from build123d import *

# Parameters (mm, degrees)
F1_DEPTH = 6.35
F2_DEPTH = 12.7


with BuildPart() as f1:
    # F0 (on Front) → F1 (new body)
    with BuildSketch(Plane.XZ):
        Polygon((-29.3310899078, 53.6682253753), (-52.3154214025, 53.6682253753), (-52.3154214025, -22.5317746247), (54.824039946, -22.5317746247), (54.824039946, -8.9082447812), (44.4758199155, -8.9082447812), (44.4758199155, -2.3659907747), (54.824039946, -2.3659907747), (54.824039946, 13.8338748366), (44.4758199155, 13.8338748366), (44.4758199155, 21.3107354939), (54.824039946, 21.3107354939), (54.824039946, 36.2644605339), (44.4758199155, 36.2644605339), (44.4758199155, 44.3643927574), (54.824039946, 44.3643927574), (54.824039946, 55.1141475241), (31.8397084513, 54.8039578557), (-29.3310899078, 53.9784150436), align=None)
    extrude(amount=F1_DEPTH)

    # F0 (on Front) → F2 (join)
    with BuildSketch(Plane.XZ):
        Polygon((-29.3310899078, 53.6682253753), (-52.3154214025, 53.6682253753), (-52.3154214025, -22.5317746247), (54.824039946, -22.5317746247), (54.824039946, -8.9082447812), (44.4758199155, -8.9082447812), (44.4758199155, -2.3659907747), (54.824039946, -2.3659907747), (54.824039946, 13.8338748366), (44.4758199155, 13.8338748366), (44.4758199155, 21.3107354939), (54.824039946, 21.3107354939), (54.824039946, 36.2644605339), (44.4758199155, 36.2644605339), (44.4758199155, 44.3643927574), (54.824039946, 44.3643927574), (54.824039946, 55.1141475241), (31.8397084513, 54.8039578557), (-29.3310899078, 53.9784150436), align=None)
        Polygon((-52.3154214025, 65.8902004361), (-52.3154214025, 53.6682253753), (-29.3310899078, 53.9784150436), (-29.3310899078, 80.5141475241), (-52.3154214025, 80.2039578557), align=None)
        Polygon((-29.3310899078, 53.9784150436), (-52.3154214025, 53.6682253753), (-29.3310899078, 53.6682253753), align=None)
        Polygon((31.8397084513, 80.2039578557), (31.8397084513, 54.8039578557), (54.824039946, 55.1141475241), (54.824039946, 80.5141475241), align=None)
        with BuildLine():
            Line((-52.3154214025, 80.2039578557), (-29.3310899078, 80.5141475241))
            ThreePointArc((-29.3310899078, 80.5141475241), (-20.5215844856, 100.1447961764), (0, 106.6127419472))
            Line((0, 106.6127419472), (0, 129.0534651811))
            ThreePointArc((0, 129.0534651811), (-36.7683139969, 115.9921461392), (-52.3154214025, 80.2039578557))
        make_face()
        with BuildLine():
            ThreePointArc((0, 106.6127419472), (22.12305543, 100.8872295472), (31.8397084513, 80.2039578557))
            Line((31.8397084513, 80.2039578557), (54.824039946, 80.5141475241))
            ThreePointArc((54.824039946, 80.5141475241), (38.3394632715, 117.1261015644), (0, 129.0534651811))
            Line((0, 129.0534651811), (0, 106.6127419472))
        make_face()
    extrude(amount=F2_DEPTH)


solid = f1.part
Geometry: final body of the model. Coordinates: model frame, mm. A direction names the side the tool comes from. Round coordinates to 2 decimals unless told otherwise and drop trailing zeros. Order: outer loops, then holes, each group sorted by start corner. A loop starts at its lowest first (then second) coordinate and runs counter-clockwise, first axis right, second up. Notation, with made-up numbers: (23.25, 23.5) -> (62.25, 23.5) arc R34 cw to (62.25, 59.5) -> close; hole circle Ø4 at (13, -26.75). An arc over 180 degrees is marked (long way). Put each result on its own line as item: value. Start each with the question number.
Q1. Section A-A on z = 71. Return the cut outline in (x, y).
Q2. Line query: probe 1 along X at (y, z) = (-4.75, 78); probe 2 along X at (y, z) = (-1, 37); probe 3 along Z at (x, y) = (20.5, -11.5). Output: solid intervals per line, ascending.
Q3. Reachability of faces 4 (the flat face through (44.476, -6, -6)), 5 (the flat face through (1, -12.7, 38)), 6 (the flat face through (31.84, -6, 68)) from +Z, -Z, +X, -X, +Y, -Y: full face, straight path, thin tool, end or side. Return the list, or none.
Q4. Section B-B on x = 27. Return the cut outline in (y, z).
Q5. First-contact query: pin 1 (5 mm diameter, centred on x = 47, y = -8, fed in from +Z); pin 2 (3.5 mm diameter, centred on y = -7, z = 17.5, fed in from +X); pin 3 (3 mm diameter, centred on x = 52, y = -5, fed in from +Z). Flat tips, straight axial feed; report the tip coordinate or a pass-through.
Q6. Section C-C on y = -4.5. Return the cut outline in (x, z).
Q7. Section D-D on x = -45. Return the cut outline in (y, z), and give its area (3 significant figures).
Q8. Pull-direction query (Z, two-part tool) for faces 1 (the flat face through (54.824, -6, -16)), 2 (the flat face through (1, -6, -22.532)), 3 (the flat face through (50, -6, 21.311)); classes: +Z half, -Z half, draft (parallel to the pull), parting line (faces both ways), or undercut.
Ans:
1. outline: (-52.32, -12.7) -> (-29.33, -12.7) -> (-29.33, 0) -> (-52.32, 0) -> close; (31.84, -12.7) -> (54.82, -12.7) -> (54.82, 0) -> (31.84, 0) -> close
2. probe 1: x = -52.32 to -29.33, 31.84 to 54.82
2. probe 2: x = -52.32 to 44.48
2. probe 3: z = -22.53 to 54.65, 102.13 to 127.19
3. face 4: +X, +Y, -Y
3. face 5: +Z, -Z, +X, -X, -Y
3. face 6: +Y, -Y
4. outline: (-12.7, -22.53) -> (0, -22.53) -> (0, 54.74) -> (-12.7, 54.74) -> close; (-12.7, 95.59) -> (0, 95.59) -> (0, 124.64) -> (-12.7, 124.64) -> close
5. pin 1: stops at z = 110.57
5. pin 2: stops at x = 44.48
5. pin 3: stops at z = 100.62
6. outline: (-52.32, -22.53) -> (54.82, -22.53) -> (54.82, -8.91) -> (44.48, -8.91) -> (44.48, -2.37) -> (54.82, -2.37) -> (54.82, 13.83) -> (44.48, 13.83) -> (44.48, 21.31) -> (54.82, 21.31) -> (54.82, 36.26) -> (44.48, 36.26) -> (44.48, 44.36) -> (54.82, 44.36) -> (54.82, 80.51) arc R48.9 ccw to (0, 129.05) arc R48.96 ccw to (-52.32, 80.2) -> close; hole (-29.33, 53.98) -> (31.84, 54.8) -> (31.84, 80.2) arc R26.87 ccw to (0, 106.61) arc R26.28 ccw to (-29.33, 80.51) -> close
7. outline: (-12.7, -22.53) -> (0, -22.53) -> (0, 105.95) -> (-12.7, 105.95) -> close
7. area: 1,630 mm2
8. face 1: draft
8. face 2: -Z half
8. face 3: undercut
